For this review, take the finished solid that the model builds, in its own axes (mm). Give positions to 0.01 mm unless a question says otherwise; leave off trailing zeros. Order: outer loops, then holes, each group sorted by start corner. A loop starts at its lowest first (then second) coordinate and runs counter-clockwise, first axis right, second up. Notation, with made-up numbers: (59.25, 7) - (102.25, 7) arc R22 ccw to (102.25, 28) - close; hole circle Ø2 at (-24, 85). An arc over 180 degrees is marked (long way). Answer as a JSON object with one key per item and string values. Group by question number.
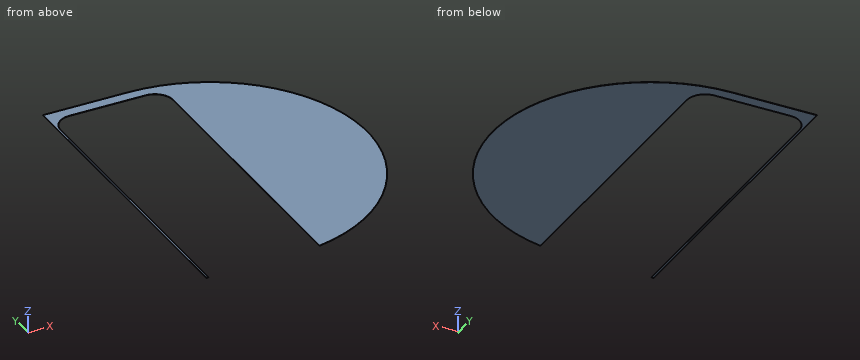
from build123d import *

# Parameters (mm, degrees)
BOSS_EXTRUDE1_DEPTH = 1
CUT_EXTRUDE2_DEPTH  = 330


with BuildPart() as part:
    # Sketch1 → Boss-Extrude1 (new body)
    with BuildSketch(Plane.XY):
        with BuildLine():
            Line((0, 0), (470, 0))
            ThreePointArc((470, 0), (1340, 870), (470, 1740))
            Line((470, 1740), (0, 1740))
            Line((0, 1740), (0, 0))
        make_face()
    extrude(amount=BOSS_EXTRUDE1_DEPTH)

    # Sketch3 → Cut-Extrude2 (cut)
    with BuildSketch(Plane(origin=(-1354.112118138, -994.457487155, -32), x_dir=(-1, 0, 0), z_dir=(0, 0, -1))):
        with BuildLine():
            Line((-1887.112118138, 819.457487155), (-1466.112118138, 819.457487155))
            ThreePointArc((-1466.112118138, 819.457487155), (-1395.40144002, 848.746809036), (-1366.112118138, 919.457487155))
            Line((-1366.112118138, 919.457487155), (-1366.112118138, 2569.457487155))
            ThreePointArc((-1366.112118138, 2569.457487155), (-1395.40144002, 2640.168165273), (-1466.112118138, 2669.457487155))
            Line((-1466.112118138, 2669.457487155), (-1887.112118138, 2669.457487155))
            ThreePointArc((-1887.112118138, 2669.457487155), (-1957.822796257, 2640.168165273), (-1987.112118138, 2569.457487155))
            Line((-1987.112118138, 2569.457487155), (-1987.112118138, 919.457487155))
            ThreePointArc((-1987.112118138, 919.457487155), (-1957.822796257, 848.746809036), (-1887.112118138, 819.457487155))
        make_face()
    extrude(amount=-CUT_EXTRUDE2_DEPTH, mode=Mode.SUBTRACT)


solid = part.part
1) Consider section A-A (y = 1007). Give the boundary of the cut face in (x, z), plus the area to 3 significant figures.
2) Consider section B-B (z = 0.45). Give the boundary of the cut face in (x, y).
3) Consider section C-C (y = 1266.5). Give the boundary of the cut face in (x, z), plus the area to 3 significant figures.
4) For line 1 (X direction, y = 865, z = 0.35); line 2 (X direction, y = 541.5, z = 0.6); line 3 (Y direction, x = 145, z = 0.55), list the stretches that pass through material, from the lowest coordinate up.
5) Consider section D-D (x = 152). Give the boundary of the cut face in (y, z), plus the area to 3 significant figures.
6) For pin 1 (0.5 mm diameter, centred on x = 396, z = 0.5, fed in from -Y), flat-tipped, find the tip position at first contact; note if it passes through.
Result set:
{
 "1": {"outline": "(0, 0) - (12, 0) - (12, 1) - (0, 1) - close; (633, 0) - (1329.15, 0) - (1329.15, 1) - (633, 1) - close", "area": "708 mm2"},
 "2": {"outline": "(0, 0) - (12, 0) - (12, 1575) arc R100 cw to (112, 1675) - (533, 1675) arc R100 cw to (633, 1575) - (633, 15.41) arc R870 ccw to (470, 1740) - (0, 1740) - close"},
 "3": {"outline": "(0, 0) - (12, 0) - (12, 1) - (0, 1) - close; (633, 0) - (1244.4, 0) - (1244.4, 1) - (633, 1) - close", "area": "623 mm2"},
 "4": {"line 1": "x = 0 to 12, 633 to 1339.99", "line 2": "x = 0 to 12, 633 to 1275.6", "line 3": "y = 1675 to 1740"},
 "5": {"outline": "(1675, 0) - (1740, 0) - (1740, 1) - (1675, 1) - close", "area": "65.0 mm2"},
 "6": {"pin 1": "stops at y = 1675"}
}
